Verification items for the finished model (mm, model axes). A direction names the side the tool comes from. Coordinates: 2 decimals unless noted, no trailing zeros. Write each loop counter-clockwise with the first axis right and the second up, starting at its lowest first coordinate (ties: lowest second). Pieces come first, ordered by that corner, then holes. Notation, with made-up numbers: (13.5, -6) - (67.5, -6) arc R4 cw to (67.5, 1) - close; hole circle Ø3 at (85, -33.5). An arc over 180 degrees is marked (long way). Answer as CSV lines item,"result". Start each with the question number.
```python
from build123d import *

# Parameters (mm, degrees)
CUT_EXTRUDE1_DEPTH      = 129.265349959
CUT_EXTRUDE1_DEPTH_BACK = 129.265349959
CUT_EXTRUDE2_DEPTH      = 129.265350019
CUT_EXTRUDE2_DEPTH_BACK = 129.265350019
SKETCH3_R               = 6


with BuildPart() as part:
    # Sketch1 → Revolve2 (revolve)
    with BuildSketch(Plane.XY, mode=Mode.PRIVATE) as revolve2_sk:
        with BuildLine():
            Line((30, 0), (40, 4))
            Line((40, 4), (40, 32))
            Line((40, 32), (72, 32))
            Line((72, 32), (72, 42))
            Line((72, 42), (40, 42))
            Line((40, 42), (40, 72))
            Line((40, 72), (34, 78))
            Line((34, 78), (0, 78))
            Line((0, 78), (0, 72))
            Line((0, 72), (33.350051409, 72))
            Line((33.350051409, 72), (33.350051409, 44.979507344))
            ThreePointArc((33.350051409, 44.979507344), (32.343772274, 42.737838966), (30, 42))
            Line((30, 42), (30, 0))
        make_face()
    revolve(revolve2_sk.sketch.rotate(Axis((0, 106.766899484, 0), (0, -1, 0)), 90), axis=Axis((0, 106.766899484, 0), (0, -1, 0)))

    # Sketch2 → Cut-Extrude1 (cut, two sides: drawn at the far end of the back side and taken through both)
    with BuildSketch(Plane(origin=(0, 78, 0), x_dir=(1, 0, 0), z_dir=(0, 1, 0)).offset(-CUT_EXTRUDE1_DEPTH_BACK)):
        with BuildLine():
            Line((-6, 23.237900077), (-6, 32))
            Line((-6, 32), (6, 32))
            Line((6, 32), (6, 23.237900077))
            ThreePointArc((6, 23.237900077), (0, -24), (-6, 23.237900077))
        make_face()
    extrude(amount=CUT_EXTRUDE1_DEPTH + CUT_EXTRUDE1_DEPTH_BACK, mode=Mode.SUBTRACT)

    # Sketch3 → Cut-Extrude2 (cut, two sides: drawn at the far end of the back side and taken through both)
    with BuildSketch(Plane(origin=(0, 78, 0), x_dir=(1, 0, 0), z_dir=(0, 1, 0)).offset(-CUT_EXTRUDE2_DEPTH_BACK)):
        with Locations(Location((0, 58, 0), (0, 0, 270))):
            Circle(SKETCH3_R)
        with Locations(Location((58, 0, 0), (0, 0, 270))):
            Circle(SKETCH3_R)
        with Locations(Location((0, -58, 0), (0, 0, 270))):
            Circle(SKETCH3_R)
        with Locations(Location((-58, 0, 0), (0, 0, 270))):
            Circle(SKETCH3_R)
    extrude(amount=CUT_EXTRUDE2_DEPTH + CUT_EXTRUDE2_DEPTH_BACK, mode=Mode.SUBTRACT)


solid = part.part
```
1. Scan lines: line 1 along X through (y, z) = (34.25, 0); line 2 along Y through (x, z) = (-55.5, 27.5); line 3 along Z through (x, y) = (-24, 57). Record each from-to range of solid material in increasing order. Write a range as from..to.
2. Depth check by flat-ended pin: P1, Ø3, axis at x = 46.5, z = -56.5, coming from the -Y side; P2, Ø3, axis at x = -9, z = 52.5, coming from the +Y side; P3, Ø1.8, axis at y = 76, z = -28.5, coming from the -X side. Enter the tip coordinate at first touch or a pass-through.
3. Access from +Z, -Z, +X, -X, +Y, -Y to the whole of each face (thin tool, end or side, straight path). Record for faces 5 (the face through (1.235, 20.706, 29.975)), 6 (the face through (-1.76, 57.21, -39.96)), 7 (the face through (0, 22, -32)).
4. Draft check along X on faces 1 (the face through (10, 72, 22)), 2 (the face through (31, 42, 31)), 3 (the face through (-1.76, 18.2, -39.96)), 4 (the face through (0, 75, -32)). Enter one of: pulls with the +X half, pulls with the -X half, needs draft (parallel to the pull), parting line crosses it, or undercut.
5. Cross-section at C-C (z = 58). Record the cut outline in (x, y), and give its area (3 significant figures).
6. Cross-section at B-B (y = 37). Record the cut outline in (x, z).
7. Cross-section at A-A (z = 0). Count the separate pieces of the cut face and the enclosed holes in it, and give its area (3 significant figures).
Completed:
1,line 1,"x = -72..-64, -52..-30, 30..52, 64..72"
1,line 2,"y = 32..42"
1,line 3,"z = -32..-23.16, 23.16..32"
2,P1,"stops at y = 32"
2,P2,"stops at y = 42"
2,P3,"stops at x = -23.8"
3,face 5,"-Y"
3,face 6,"+Y"
3,face 7,"+Y, -Y"
4,face 1,"undercut"
4,face 2,"needs draft"
4,face 3,"parting line crosses it"
4,face 4,"undercut"
5,outline,"(-42.66, 32) - (-6, 32) - (-6, 42) - (-42.66, 42) - close; (6, 32) - (42.66, 32) - (42.66, 42) - (6, 42) - close"
5,area,"733 mm2"
6,outline,"circle Ø144 at (0, 0); hole circle Ø12 at (-58, 0); hole circle Ø12 at (0, -58); hole (-6, -32) - (6, -32) - (6, -29.39) arc R30 ccw (long way) to (-6, -29.39) - close; hole circle Ø12 at (0, 58); hole circle Ø12 at (58, 0)"
7,separate pieces,"4"
7,enclosed holes,"0"
7,area,"1,760 mm2"
